Verification items for the finished model (mm, model axes). A direction names the side the tool comes from. Give positions to 0.01 mm unless a question says otherwise; leave off trailing zeros. Write each loop counter-clockwise with the first axis right and the second up, starting at its lowest first coordinate (ties: lowest second). Pieces come first, ordered by that corner, then holes. Notation, with made-up numbers: (11, 56) -> (35, 56) arc R27 cw to (35, 77) -> close; hole circle Ø7 at (70, -19). An arc over 180 degrees is marked (long way). Use CSV: the item, a comma, the result in double quotes. Start each with the question number.
```python
from build123d import *

# Parameters (mm, degrees)
BOSS_EXTRUDE1_DEPTH = 2
BOSS_EXTRUDE2_DEPTH = 2
CUT_EXTRUDE1_REACH  = 34.818
SKETCH4_R           = 4.5
SKETCH4_R_2         = 1.4
CUT_EXTRUDE2_REACH  = 34.818
SKETCH5_R           = 1.6


with BuildPart() as part:
    # Sketch2 → Boss-Extrude1 (new body)
    with BuildSketch(Plane.XY):
        with BuildLine():
            Line((-27, -10), (27, -10))
            ThreePointArc((27, -10), (29.828427125, -8.828427125), (31, -6))
            Line((31, -6), (31, 6))
            ThreePointArc((31, 6), (29.828427125, 8.828427125), (27, 10))
            Line((27, 10), (-27, 10))
            ThreePointArc((-27, 10), (-29.828427125, 8.828427125), (-31, 6))
            Line((-31, 6), (-31, -6))
            ThreePointArc((-31, -6), (-29.828427125, -8.828427125), (-27, -10))
        make_face()
    extrude(amount=BOSS_EXTRUDE1_DEPTH)

    # Sketch3 → Boss-Extrude2 (add)
    with BuildSketch(Plane.XY.offset(2)):
        with BuildLine():
            Line((-28.585786438, 1.414213562), (-23, 7))
            Line((-23, 7), (23, 7))
            Line((23, 7), (28.585786438, 1.414213562))
            ThreePointArc((28.585786438, 1.414213562), (29.171572875, 0), (28.585786438, -1.414213562))
            Line((28.585786438, -1.414213562), (23, -7))
            Line((23, -7), (22, -7))
            ThreePointArc((22, -7), (20.585786438, -7.585786438), (20, -9))
            Line((20, -9), (20, -10))
            Line((20, -10), (-20, -10))
            Line((-20, -10), (-20, -9))
            ThreePointArc((-20, -9), (-20.585786438, -7.585786438), (-22, -7))
            Line((-22, -7), (-23, -7))
            Line((-23, -7), (-28.585786438, -1.414213562))
            ThreePointArc((-28.585786438, -1.414213562), (-29.171572875, 0), (-28.585786438, 1.414213562))
        make_face()
    extrude(amount=BOSS_EXTRUDE2_DEPTH)

    # Sketch4 → Cut-Extrude1 (cut, up to next)
    with BuildSketch(Plane(origin=(0, 0, 0), x_dir=(-1, 0, 0), z_dir=(0, 0, -1)), mode=Mode.PRIVATE) as cut_extrude1_sk1:
        Circle(SKETCH4_R)
    cut_extrude1_tool1 = extrude(cut_extrude1_sk1.sketch, amount=-CUT_EXTRUDE1_REACH, mode=Mode.PRIVATE) & part.part
    # Sketch4 → Cut-Extrude1 (cut, up to next)
    with BuildSketch(Plane(origin=(0, 0, 0), x_dir=(-1, 0, 0), z_dir=(0, 0, -1)), mode=Mode.PRIVATE) as cut_extrude1_sk2:
        with Locations((-18.5, 0)):
            Circle(SKETCH4_R_2)
    cut_extrude1_tool2 = extrude(cut_extrude1_sk2.sketch, amount=-CUT_EXTRUDE1_REACH, mode=Mode.PRIVATE) & part.part
    # Sketch4 → Cut-Extrude1 (cut, up to next)
    with BuildSketch(Plane(origin=(0, 0, 0), x_dir=(-1, 0, 0), z_dir=(0, 0, -1)), mode=Mode.PRIVATE) as cut_extrude1_sk3:
        with Locations(Location((18.5, 0, 0), (0, 0, 180))):
            Circle(SKETCH4_R_2)
    cut_extrude1_tool3 = extrude(cut_extrude1_sk3.sketch, amount=-CUT_EXTRUDE1_REACH, mode=Mode.PRIVATE) & part.part
    add(cut_extrude1_tool1.solids().sort_by_distance((0, 0, 0))[0], mode=Mode.SUBTRACT)
    add(cut_extrude1_tool2.solids().sort_by_distance((18.5, 0, 0))[0], mode=Mode.SUBTRACT)
    add(cut_extrude1_tool3.solids().sort_by_distance((-18.5, 0, 0))[0], mode=Mode.SUBTRACT)

    # Sketch5 → Cut-Extrude2 (cut, up to next)
    with BuildSketch(Plane(origin=(0, 0, 0), x_dir=(-1, 0, 0), z_dir=(0, 0, -1)), mode=Mode.PRIVATE) as cut_extrude2_sk1:
        with Locations((-27, 7)):
            Circle(SKETCH5_R)
    cut_extrude2_tool1 = extrude(cut_extrude2_sk1.sketch, amount=-CUT_EXTRUDE2_REACH, mode=Mode.PRIVATE) & part.part
    # Sketch5 → Cut-Extrude2 (cut, up to next)
    with BuildSketch(Plane(origin=(0, 0, 0), x_dir=(-1, 0, 0), z_dir=(0, 0, -1)), mode=Mode.PRIVATE) as cut_extrude2_sk2:
        with Locations((27, 7)):
            Circle(SKETCH5_R)
    cut_extrude2_tool2 = extrude(cut_extrude2_sk2.sketch, amount=-CUT_EXTRUDE2_REACH, mode=Mode.PRIVATE) & part.part
    # Sketch5 → Cut-Extrude2 (cut, up to next)
    with BuildSketch(Plane(origin=(0, 0, 0), x_dir=(-1, 0, 0), z_dir=(0, 0, -1)), mode=Mode.PRIVATE) as cut_extrude2_sk3:
        with Locations((27, -7)):
            Circle(SKETCH5_R)
    cut_extrude2_tool3 = extrude(cut_extrude2_sk3.sketch, amount=-CUT_EXTRUDE2_REACH, mode=Mode.PRIVATE) & part.part
    # Sketch5 → Cut-Extrude2 (cut, up to next)
    with BuildSketch(Plane(origin=(0, 0, 0), x_dir=(-1, 0, 0), z_dir=(0, 0, -1)), mode=Mode.PRIVATE) as cut_extrude2_sk4:
        with Locations((-27, -7)):
            Circle(SKETCH5_R)
    cut_extrude2_tool4 = extrude(cut_extrude2_sk4.sketch, amount=-CUT_EXTRUDE2_REACH, mode=Mode.PRIVATE) & part.part
    add(cut_extrude2_tool1.solids().sort_by_distance((27, 7, 0))[0], mode=Mode.SUBTRACT)
    add(cut_extrude2_tool2.solids().sort_by_distance((-27, 7, 0))[0], mode=Mode.SUBTRACT)
    add(cut_extrude2_tool3.solids().sort_by_distance((-27, -7, 0))[0], mode=Mode.SUBTRACT)
    add(cut_extrude2_tool4.solids().sort_by_distance((27, -7, 0))[0], mode=Mode.SUBTRACT)


solid = part.part
```
(1) Draft check along Y on faces 4 (the face through (20.6, -7.57, 2.99)), 5 (the face through (-26, 4, 3)), 6 (the face through (28.27, -7.97, 0.99)), 7 (the face through (-20, -9.5, 3)). Enter one of: released by +Y, released by -Y, zero draft, split by the parting line, or undercut.
(2) Section check B-B on y = -3.5. Record the cut outline in (x, z).
(3) Section check C-C on x = 0. Record the cut outline in (y, z), then the cut area to 3 significant figures.
(4) Go/stop test with flat-tipped pins: pin 1 (0.5 mm diameter, centred on y = -9.5, z = 3.5, fed in from +X); pin 2 (1.1 mm diameter, centred on x = -22.5, z = 3.5, fed in from -Y); pin 3 (0.6 mm diameter, centred on x = -8, z = 3.5, fed in from +Y). Record where each tip stops, or that it passes through.
(5) Set-up check for faces 1 (the face through (-2.4, 7.5, 2)), 2 (the face through (-29.17, -0.02, 2.99)), 3 (the face through (29.17, 0.02, 2.99)): record each of +Z, -Z, +X, -X, +Y, -Y from which the full face is reachable in a straight line by a thin tool's end or side.
(6) Section check A-A on x = 18.5. Record the cut outline in (y, z), then the cut area to 3 significant figures.
(7) Thickness scan on line 1 (Y direction, x = -27, z = 1.25); line 2 (Y direction, x = -18.5, z = 2.2); line 3 (X direction, y = -6.25, z = 0.8). Record the ranges inside material, lowest first. Write a range as from..to.
Data:
1,face 4,"released by -Y"
1,face 5,"released by +Y"
1,face 6,"undercut"
1,face 7,"zero draft"
2,outline,"(-31, 0) -> (-2.83, 0) -> (-2.83, 4) -> (-26.5, 4) -> (-26.5, 2) -> (-31, 2) -> close; (2.83, 0) -> (31, 0) -> (31, 2) -> (26.5, 2) -> (26.5, 4) -> (2.83, 4) -> close"
3,outline,"(-10, 0) -> (-4.5, 0) -> (-4.5, 4) -> (-10, 4) -> close; (4.5, 0) -> (10, 0) -> (10, 2) -> (7, 2) -> (7, 4) -> (4.5, 4) -> close"
3,area,"38.0 mm2"
4,pin 1,"stops at x = 20"
4,pin 2,"stops at y = -7"
4,pin 3,"stops at y = 7"
5,face 1,"+Z"
5,face 2,"+Z, -X"
5,face 3,"+Z, +X"
6,outline,"(-10, 0) -> (-1.4, 0) -> (-1.4, 4) -> (-10, 4) -> close; (1.4, 0) -> (10, 0) -> (10, 2) -> (7, 2) -> (7, 4) -> (1.4, 4) -> close"
6,area,"62.8 mm2"
7,line 1,"y = -10..-8.6, -5.4..5.4, 8.6..10"
7,line 2,"y = -10..-1.4, 1.4..7"
7,line 3,"x = -30.99..-28.41, -25.59..25.59, 28.41..30.99"
